Geometry: final body of the model. Coordinates: model frame, mm. A direction names the side the tool comes from. Give positions to 0.01 mm unless a question says otherwise; leave off trailing zeros. Write each loop counter-clockwise with the first axis right and the second up, starting at its lowest first coordinate (ties: lowest second). Pieces come first, ordered by that corner, then holes.
from build123d import *

# Parameters (mm, degrees)
F0_R           = 4.4323867957
F1_DEPTH       = 5.08
F1_DEPTH_BACK  = 38.1
F1_FACE_R      = 4.4323867957
F2_DEPTH       = 2.54
F2_TAPER       = 10
F1_FACE1_R     = 4.4323867957
F3_DEPTH       = 2.54
F3_TAPER       = 10
F4_R           = 1.7950151947
F5_DEPTH       = 2.54
F5_TAPER       = -20
F6_R           = 2.6311933972
F7_DEPTH       = 2.54
F7_TAPER       = 20
F8_W           = 1.8805181608
F8_H           = 6.0816761106
F9_DEPTH       = 25.4
F9_DEPTH_BACK  = 25.4
F10_W          = 1.8878498813
F10_H          = 6.0830730945
F11_DEPTH      = 25.4
F11_DEPTH_BACK = 25.4


with BuildPart() as f1:
    # F0 (on Top) → F1 (new body, two sides)
    with BuildSketch(Plane.XY) as f1_sk:
        Circle(F0_R)
    extrude(amount=F1_DEPTH)
    extrude(f1_sk.sketch, amount=-F1_DEPTH_BACK)

    # F1_face (on face) → F2 (join)
    with BuildSketch(Plane(origin=(0, 0, -38.1), x_dir=(1, 0, 0), z_dir=(0, 0, -1))):
        Circle(F1_FACE_R)
    extrude(amount=F2_DEPTH, taper=F2_TAPER)

    # F1_face1 (on face) → F3 (join)
    with BuildSketch(Plane.XY.offset(5.08)):
        Circle(F1_FACE1_R)
    extrude(amount=F3_DEPTH, taper=F3_TAPER)

    # F4 (on face) → F5 (join)
    with BuildSketch(Plane(origin=(0, 0, -40.64), x_dir=(1, 0, 0), z_dir=(0, 0, -1))):
        Circle(F4_R)
    extrude(amount=F5_DEPTH, taper=F5_TAPER)

    # F6 (on face) → F7 (cut)
    with BuildSketch(Plane(origin=(0, 0, -43.18), x_dir=(1, 0, 0), z_dir=(0, 0, -1))):
        Circle(F6_R)
    extrude(amount=-F7_DEPTH, taper=F7_TAPER, mode=Mode.SUBTRACT)

    # F8 (on Right) → F9 (cut, two sides)
    with BuildSketch(Plane.YZ) as f9_sk:
        with Locations((-0.0123365317, -33.8487112895)):
            Rectangle(F8_W, F8_H)
    extrude(amount=-F9_DEPTH, mode=Mode.SUBTRACT)
    extrude(f9_sk.sketch, amount=F9_DEPTH_BACK, mode=Mode.SUBTRACT)

    # F10 (on Front) → F11 (cut, two sides)
    with BuildSketch(Plane.XZ) as f11_sk:
        with Locations((-0.0861281878, -33.9269181713)):
            Rectangle(F10_W, F10_H)
    extrude(amount=-F11_DEPTH, mode=Mode.SUBTRACT)
    extrude(f11_sk.sketch, amount=F11_DEPTH_BACK, mode=Mode.SUBTRACT)


solid = f1.part
Q1. Section A-A on z = -36. Output: boundary loops of the cut face in (x, y).
Filled sheet:
outline: (-4.33, -0.95) arc R4.43 ccw to (-1.03, -4.31) - (-1.03, -0.95) - close; (-4.33, 0.93) - (-1.03, 0.93) - (-1.03, 4.31) arc R4.43 ccw to start; (0.86, -4.35) arc R4.43 ccw to (4.33, -0.95) - (0.86, -0.95) - close; (0.86, 0.93) - (4.33, 0.93) arc R4.43 ccw to (0.86, 4.35) - close
Q2. Access query for faces 1 (the flat face through (2, -0.953, -34)), 2 (the flat face through (0, -3, -30.885)), 3 (the flat face through (2, 1, -40.64)), 4 (the conical face through (3.87, -1.22, -40.23)). Directions: +Z, -Z, +X, -X, +Y, -Y. A direction counts if a zero-diameter tool reaches every point of the face in a straight line with its end or side. Return the directions, or none.
Filled sheet:
face 1: +X, -X
face 2: +Y, -Y
face 3: none
face 4: -Z
Q3. Pin query (flat end, axial travel): P1, Ø2.5, axis at x = 0, y = 0, coming from the -Z side; P2, Ø3, axis at y = 2, z = -34.5, coming from the +X side; P3, Ø1.5, axis at x = -1, z = -37, coming from the -Y side. Return the tip coordinate at first contact, or that it passes through.
Filled sheet:
P1: stops at z = -40.64
P2: stops at x = 4.33
P3: stops at y = -4.43
Q4. Section C-C on z = -2. Output: boundary loops of the cut face in (x, y).
Filled sheet:
outline: circle Ø8.86 at (0, 0)
Q5. Pull-direction query (Z, two-part tool) for faces 5 (the conical face through (3.87, 1.22, 7.21)), 6 (the flat face through (3, 0, -36.89)), 7 (the flat face through (0, 0, -40.64)); classes: released by +Z, released by -Z, zero draft, split by the parting line, or undercut.
Filled sheet:
face 5: released by +Z
face 6: undercut
face 7: released by -Z
Q6. Ray query, line 1 along Z through (x, y) = (-2.75, 0.25); line 2 along Y through (x, z) = (1, -29); line 3 along X through (y, z) = (3.5, -10). Return the intervals inside material, ascending.
Filled sheet:
line 1: z = -40.64 to -36.89, -30.81 to 7.62
line 2: y = -4.32 to 4.32
line 3: x = -2.72 to 2.72
Q7. Section B-B on x = 0. Output: boundary loops of the cut face in (y, z), plus the area to 3 significant figures.
Filled sheet:
outline: (-4.43, -38.1) - (-3.98, -40.64) - (-1.8, -40.64) - (-2.72, -43.18) - (-2.63, -43.18) - (-1.71, -40.64) - (1.71, -40.64) - (2.63, -43.18) - (2.72, -43.18) - (1.8, -40.64) - (3.98, -40.64) - (4.43, -38.1) - (4.43, -36.97) - (-4.43, -36.97) - close; (-4.43, -30.89) - (-0.95, -30.89) - (-0.95, -30.81) - (0.93, -30.81) - (0.93, -30.89) - (4.43, -30.89) - (4.43, 5.08) - (3.98, 7.62) - (-3.98, 7.62) - (-4.43, 5.08) - close
area: 372 mm2
